Verification items for this drawing (mm, ordinates from the low corner). Round coordinates to 2 decimals unless told otherwise and drop trailing zeros. Order: outer loops, then holes, each group sorted by start corner. A loop starts at its lowest first (then second) coordinate and runs counter-clockwise, first axis right, second up. Notation, with made-up numbers: (-10.5, 86.5) - (46.5, 86.5) arc R21 ccw to (46.5, 111.5) - close; hole circle Ø2 at (69, 31). An arc over 180 degrees is marked (long way). Return JSON: item names as keys, results as strings. Group by question number.
Q1. Sectioned sample at A-A, the plane y = 35. Record the cut outline in (x, z).
Q2. Sectioned sample at C-C, the plane x = 8. Record the cut outline in (y, z).
Q3. Gauge pin test, flat ends, axial feed: pin 1 Ø12 at (y, z) = (15, 76) entering from -X; pin 2 Ø4 at (x, z) = (10, 53.5) entering from +Y. Record the tip position at first contact, or that the pin passes through.
Q4. Material ranges on line 1 along Z through (x, y) = (2.3, 35); line 2 along Y through (x, z) = (2.95, 5); line 3 along X through (y, z) = (35.5, 73), recorded low to high.
Q5. Draft check along X on the marked faces 1, 2, 3 and 4. Enter one of: pulls with the +X half, pulls with the -X half, needs draft (parallel to the pull), parting line crosses it, or undercut.
Q6. Sectioned sample at B-B, the plane z = 115. Record the cut outline in (x, y), then the cut area to 3 significant figures.
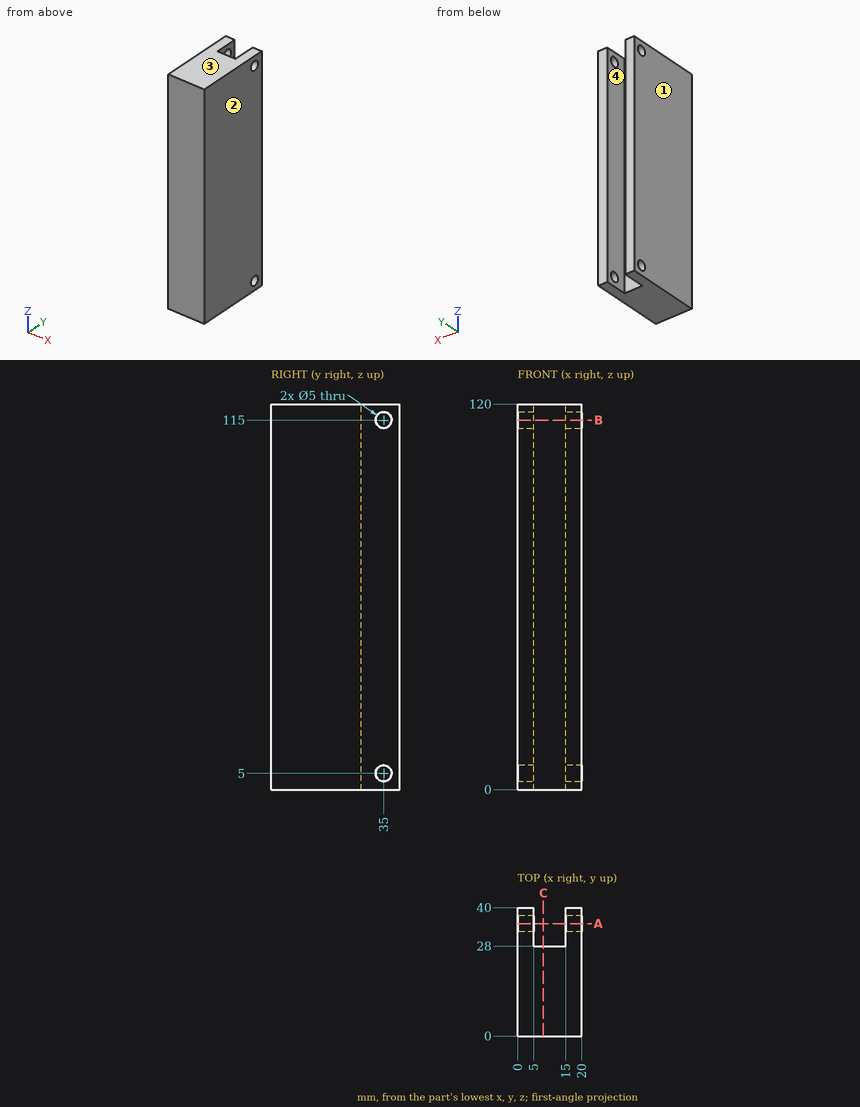
Reply:
{
 "1": {"outline": "(0, 0) - (5, 0) - (5, 2.5) - (0, 2.5) - close; (0, 7.5) - (5, 7.5) - (5, 112.5) - (0, 112.5) - close; (0, 117.5) - (5, 117.5) - (5, 120) - (0, 120) - close; (15, 0) - (20, 0) - (20, 2.5) - (15, 2.5) - close; (15, 7.5) - (20, 7.5) - (20, 112.5) - (15, 112.5) - close; (15, 117.5) - (20, 117.5) - (20, 120) - (15, 120) - close"},
 "2": {"outline": "(0, 0) - (28, 0) - (28, 120) - (0, 120) - close"},
 "3": {"pin 1": "x = 0", "pin 2": "y = 28"},
 "4": {"line 1": "0 to 2.5, 7.5 to 112.5, 117.5 to 120", "line 2": "0 to 32.5, 37.5 to 40", "line 3": "0 to 5, 15 to 20"},
 "5": {"face 1": "pulls with the -X half", "face 2": "pulls with the +X half", "face 3": "needs draft", "face 4": "undercut"},
 "6": {"outline": "(0, 0) - (20, 0) - (20, 32.5) - (15, 32.5) - (15, 28) - (5, 28) - (5, 32.5) - (0, 32.5) - close; (0, 37.5) - (5, 37.5) - (5, 40) - (0, 40) - close; (15, 37.5) - (20, 37.5) - (20, 40) - (15, 40) - close", "area": "630 mm^2"}
}
